```python
from build123d import *

# Parameters (mm, degrees)
ESQUISSE1_R             = 5.95
BOSS_EXTRU_1_DEPTH      = 75
ESQUISSE2_W             = 3.1
ESQUISSE2_H             = 3.1
ENL_V_MAT_EXTRU_1_DEPTH = 76.470557173


with BuildPart() as part:
    # Esquisse1 → Boss.-Extru.1 (new body)
    with BuildSketch(Plane.XY):
        Circle(ESQUISSE1_R)
    extrude(amount=BOSS_EXTRU_1_DEPTH)

    # Esquisse2 → Enlèv. mat.-Extru.1 (cut, through all)
    with BuildSketch(Plane(origin=(0, 0, 0), x_dir=(-1, 0, 0), z_dir=(0, 0, -1))):
        Rectangle(ESQUISSE2_W, ESQUISSE2_H)
    extrude(amount=-ENL_V_MAT_EXTRU_1_DEPTH, mode=Mode.SUBTRACT)


solid = part.part
```
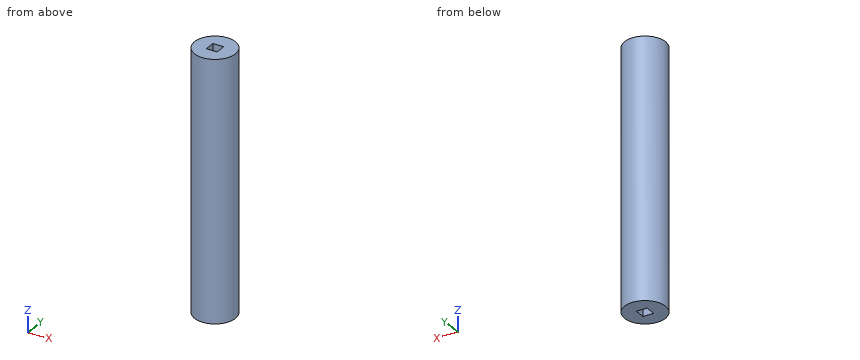
Geometry check sheet. Reference: the model listing, model coordinates, mm. Round coordinates to 2 decimals unless told otherwise and drop trailing zeros. Order: outer loops, then holes, each group sorted by start corner. A loop starts at its lowest first (then second) coordinate and runs counter-clockwise, first axis right, second up. Notation, with made-up numbers: (-29, 9) -> (5, 9) arc R8 ccw to (5, 15) -> close; hole circle Ø7 at (-0.5, 38.5). An arc over 180 degrees is marked (long way). Return JSON: item names as keys, results as strings. Group by question number.
Q1. Gauge pin test, flat end, axial feed: pin 1 (4 mm diameter, centred on y = -3.5, z = 51.5, fed in from +X). Record the tip position at first contact, or that the pin passes through.
Q2. Section check D-D, the plane y = -4.25. Record the boundary of the cut face in (x, z), plus the area to 3 significant figures.
Q3. Section check C-C, the plane z = 31. Record the boundary of the cut face in (x, y).
Q4. Section check A-A, the plane x = 0. Record the boundary of the cut face in (y, z), plus the area to 3 significant figures.
Q5. Material ranges on probe 1 along Y at (x, z) = (-0.5, 21.5); probe 2 along X at (y, z) = (0.25, 20); probe 3 along Y at (x, z) = (1.5, 64), recorded low to high. Write a range as from..to.
Numbers:
{
 "1": {"pin 1": "x = 5.76"},
 "2": {"outline": "(-4.16, 0) -> (4.16, 0) -> (4.16, 75) -> (-4.16, 75) -> close", "area": "625 mm^2"},
 "3": {"outline": "circle Ø11.9 at (0, 0); hole (-1.55, -1.55) -> (1.55, -1.55) -> (1.55, 1.55) -> (-1.55, 1.55) -> close"},
 "4": {"outline": "(-5.95, 0) -> (-1.55, 0) -> (-1.55, 75) -> (-5.95, 75) -> close; (1.55, 0) -> (5.95, 0) -> (5.95, 75) -> (1.55, 75) -> close", "area": "660 mm^2"},
 "5": {"probe 1": "-5.93..-1.55, 1.55..5.93", "probe 2": "-5.94..-1.55, 1.55..5.94", "probe 3": "-5.76..-1.55, 1.55..5.76"}
}
